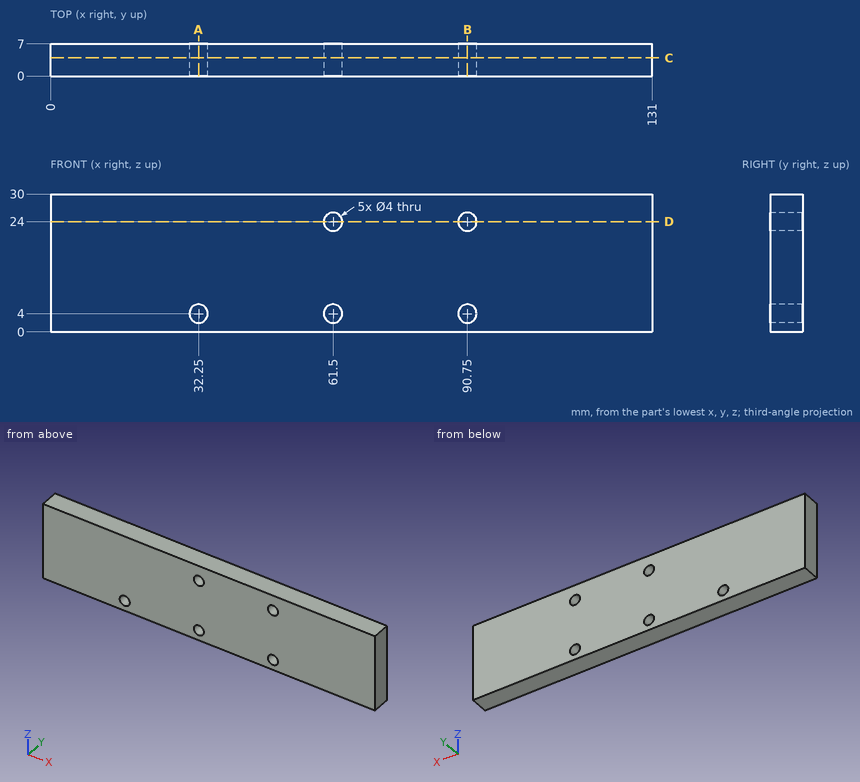
Print and shaded views of the part. All mm, measured from the part's lowest x, y and z. Coordinates: 2 decimals unless noted, no trailing zeros. Order: outer loops, then holes, each group sorted by start corner. A loop starts at its lowest first (then second) coordinate and runs counter-clockwise, first axis right, second up. Notation, with made-up numbers: (80, -3) -> (112, -3) arc R22 cw to (112, 36) -> close; hole circle Ø10 at (56, -21). An arc over 180 degrees is marked (long way). Answer as a JSON object with one key per item and string values. Group by question number.
1) Cut at D-D, the plane z = 24. Write the cut outline in (x, y).
2) Cut at B-B, the plane x = 90.75. Write the cut outline in (y, z), then the cut area to 3 significant figures.
3) Drill centre lines: L1, parallel to Z at x = 90.75, y = 3.25; L2, parallel to X at y = 6, z = 3; L3, parallel to Z at x = 32.25, y = 5. Where is each one in solid material? Low to high.
4) Cut at C-C, the plane y = 4. Write the cut outline in (x, z), then the cut area to 3 significant figures.
5) Cut at A-A, the plane x = 32.25. Write the cut outline in (y, z).
6) Flat gauge pin, fed straight in: pin 1 (3.5 mm diameter, centred on x = 90.75, z = 4, fed in from -Y). Where does the tip first touch, or does it go through?
Check values:
{
 "1": {"outline": "(0, 0) -> (59.5, 0) -> (59.5, 7) -> (0, 7) -> close; (63.5, 0) -> (88.75, 0) -> (88.75, 7) -> (63.5, 7) -> close; (92.75, 0) -> (131, 0) -> (131, 7) -> (92.75, 7) -> close"},
 "2": {"outline": "(0, 0) -> (7, 0) -> (7, 2) -> (0, 2) -> close; (0, 6) -> (7, 6) -> (7, 22) -> (0, 22) -> close; (0, 26) -> (7, 26) -> (7, 30) -> (0, 30) -> close", "area": "154 mm²"},
 "3": {"L1": "z = 0 to 2, 6 to 22, 26 to 30", "L2": "x = 0 to 30.52, 33.98 to 59.77, 63.23 to 89.02, 92.48 to 131", "L3": "z = 0 to 2, 6 to 30"},
 "4": {"outline": "(0, 0) -> (131, 0) -> (131, 30) -> (0, 30) -> close; hole circle Ø4 at (32.25, 4); hole circle Ø4 at (61.5, 4); hole circle Ø4 at (61.5, 24); hole circle Ø4 at (90.75, 4); hole circle Ø4 at (90.75, 24)", "area": "3,870 mm²"},
 "5": {"outline": "(0, 0) -> (7, 0) -> (7, 2) -> (0, 2) -> close; (0, 6) -> (7, 6) -> (7, 30) -> (0, 30) -> close"},
 "6": {"pin 1": "passes through"}
}
